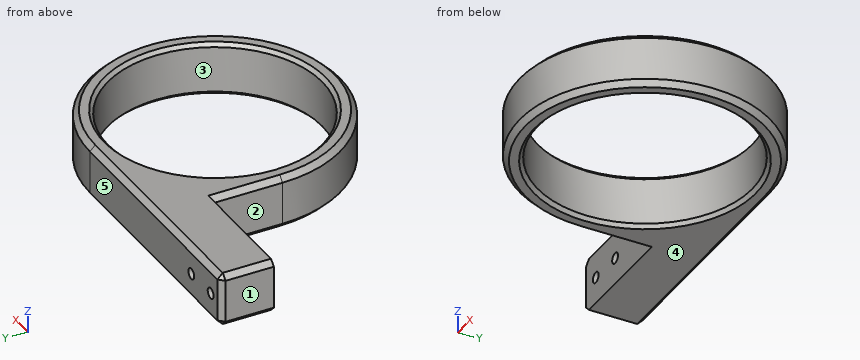
```python
from build123d import *

# Parameters (mm, degrees)
SKETCH_1_R           = 35
EXTRUDE_1_DEPTH      = 15
SKETCH_2_R           = 30
CUT_EXTRUDE_1_DEPTH  = 52.720402164
EXTRUDE_2_REACH      = 81.687
EXTRUDE_2_END_RADIUS = 35
SKETCH_3_W           = 15
SKETCH_3_H           = 15
SKETCH_4_W           = 15
SKETCH_4_H           = 15
EXTRUDE_3_DEPTH      = 32.5
EXTRUDE_4_REACH      = 81.687
SKETCH_6_W           = 15
SKETCH_6_H           = 20
SKETCH_7_R           = 1.5
CUT_EXTRUDE_2_DEPTH  = 89.352985235
CHAMFER_1_SIZE       = 1
CHAMFER_2_SIZE       = 1.5


with BuildPart() as part:
    # 草图1 → 凸台-拉伸1 (new body)
    with BuildSketch(Plane.XY):
        Circle(SKETCH_1_R)
    extrude(amount=EXTRUDE_1_DEPTH)

    # 草图2 → 切除-拉伸1 (cut, through all)
    with BuildSketch(Plane(origin=(0, 0, 0), x_dir=(-1, 0, 0), z_dir=(0, 0, -1))):
        Circle(SKETCH_2_R)
    extrude(amount=-CUT_EXTRUDE_1_DEPTH, mode=Mode.SUBTRACT)

    # 凸台-拉伸2: up to this cylinder (the profile starts outside it)
    extrude_2_end = Plane(origin=(0, 0, 7.5), z_dir=(0, 0, -1)) * Cylinder(EXTRUDE_2_END_RADIUS, 234.374, mode=Mode.PRIVATE)
    # 草图3 → 凸台-拉伸2 (add, up to the surface)
    with BuildSketch(Plane.ZY.offset(35), mode=Mode.PRIVATE) as extrude_2_sk1:
        with Locations((7.5, 27.5)):
            Rectangle(SKETCH_3_W, SKETCH_3_H)
    extrude_2_tool1 = extrude(extrude_2_sk1.sketch, amount=-EXTRUDE_2_REACH, mode=Mode.PRIVATE) - extrude_2_end
    add(extrude_2_tool1.solids().sort_by_distance((-35, 27.5, 7.5))[0])

    # 草图4 → 凸台-拉伸3 (add)
    with BuildSketch(Plane.ZY.offset(35)):
        with Locations((7.5, 27.5)):
            Rectangle(SKETCH_4_W, SKETCH_4_H)
    extrude(amount=EXTRUDE_3_DEPTH)

    # 草图6 → 凸台-拉伸4 (add, up to next)
    with BuildSketch(Plane.ZY.offset(35), mode=Mode.PRIVATE) as extrude_4_sk1:
        with Locations((7.5, 10)):
            Rectangle(SKETCH_6_W, SKETCH_6_H)
    extrude_4_tool1 = extrude(extrude_4_sk1.sketch, amount=-EXTRUDE_4_REACH, mode=Mode.PRIVATE) - part.part
    add(extrude_4_tool1.solids().sort_by_distance((-35, 10, 7.5))[0])

    # 草图7 → 切除-拉伸2 (cut, through all)
    with BuildSketch(Plane.XZ.offset(-20)):
        with Locations(Location((-62.5, 7.5, 0), (0, 0, 270))):
            Circle(SKETCH_7_R)
        with Locations(Location((-52.5, 7.5, 0), (0, 0, 270))):
            Circle(SKETCH_7_R)
    extrude(amount=-CUT_EXTRUDE_2_DEPTH, mode=Mode.SUBTRACT)

    # 倒角1
    chamfer_1_edges = [part.edges().sort_by_distance(p)[0] for p in [
        (30, 0, 15),
        (30, 0, 0),
    ]]
    chamfer(chamfer_1_edges, length=CHAMFER_1_SIZE)

    # 倒角2
    chamfer_2_edges = [part.edges().sort_by_distance(p)[0] for p in [
        (-33.75, 35, 15),
        (-33.75, 35, 0),
        (-67.5, 27.5, 0),
        (-67.5, 27.5, 15),
        (-67.5, 35, 7.5),
        (24.748737342, -24.748737342, 0),
        (24.748737342, -24.748737342, 15),
        (-35, 10, 0),
        (-35, 10, 15),
    ]]
    chamfer(chamfer_2_edges, length=CHAMFER_2_SIZE)


solid = part.part
```
Geometry: final body of the model. Coordinates: model frame, mm. Face numbers are marked on the shaded views. A direction names the side the tool comes from. Round coordinates to 2 decimals unless told otherwise and drop trailing zeros. Write each loop counter-clockwise with the first axis right and the second up, starting at its lowest first coordinate (ties: lowest second). Pieces come first, ordered by that corner, then holes.
Item 1: Section query C-C (y = 23.5). Give the number of separate pieces and of enclosed holes in the cut face, plus the area to 3 significant figures.
Item 2: Mould query, pull axis Y, two halves, no side actions, for the marked faces 3, 4 and 5. Classes: +Y half, -Y half, draft (parallel to the pull), parting line (faces both ways), or undercut.
Item 3: Section query B-B (z = 7.5). Return loops of the section in (x, y).
Item 4: Section query A-A (x = -52.5). Return loops of the section in (y, z), plus the area to 3 significant figures.
Item 5: Pin query (flat end, axial travel): P1, Ø1, axis at y = -25.5, z = 12, coming from the -X side; P2, Ø3.5, axis at y = 7, z = 8.5, coming from the -X side; P3, Ø3, axis at y = -23.5, z = 8.5, coming from the -X side. Return the tip coordinate at first contact, or that it passes through.
Item 6: Set-up query: the marked faces 1 and 2. Return all of +Z, -Z, +X, -X, +Y, -Y with unobstructed straight access to the full face (end or side cutting, diameter ignored); none if empty.
Item 7: Material intervals for L1, parallel to Y at x = 0, z = 10.25; L2, parallel to X at y = 24.5, z = 7.5 (3 decimals); L3, parallel to Z at x = -52, y = 31, sorted ascending.
Completed:
1. separate pieces: 2
1. enclosed holes: 2
1. area: 819 mm2
2. face 3: undercut
2. face 4: draft
2. face 5: +Y half
3. outline: (-67.5, 20) - (-64, 20) - (-64, 35) - (-66, 35) - (-67.5, 33.5) - close; (-61, 20) - (-54, 20) - (-54, 35) - (-61, 35) - close; (-51, 20) - (-35, 20) - (-35, 0) arc R35 ccw (long way) to (0, 35) - (-51, 35) - close; hole circle Ø60 at (0, 0)
4. outline: (20, 0) - (33.5, 0) - (35, 1.5) - (35, 6) - (20, 6) - close; (20, 9) - (35, 9) - (35, 13.5) - (33.5, 15) - (20, 15) - close
4. area: 178 mm2
5. P1: stops at x = -24.49
5. P2: stops at x = -35
5. P3: stops at x = -27.22
6. face 1: +Z, -Z, -X, +Y, -Y
6. face 2: +Z, -Z, -X, -Y
7. L1: y = -35 to -30, 30 to 35
7. L2: x = -67.5 to -64, -61 to -54, -51 to -17.313, 17.313 to 24.995
7. L3: z = 0 to 6.09, 8.91 to 15
